from build123d import *

# Parameters (mm, degrees)
SKETCH_1_W          = 120
SKETCH_1_H          = 20
EXTRUDE_1_DEPTH     = 50
SKETCH_2_W          = 6
SKETCH_2_H          = 20
EXTRUDE_2_DEPTH     = 20
CUT_EXTRUDE_1_DEPTH = 114
SKETCH_4_R          = 2.6
SKETCH_4_W          = 20
SKETCH_4_H          = 20
CUT_EXTRUDE_2_DEPTH = 114
SKETCH_5_R          = 5
CUT_EXTRUDE_3_DEPTH = 3
CUT_EXTRUDE_4_DEPTH = 300
SKETCH_8_R          = 5
CUT_EXTRUDE_5_DEPTH = 300
SKETCH_9_R          = 5
SKETCH_9_R_2        = 2.6
EXTRUDE_3_DEPTH     = 3


with BuildPart() as part:
    # 草图1 → 凸台-拉伸1 (new body)
    with BuildSketch(Plane(origin=(0, 0, 0), x_dir=(1, 0, 0), z_dir=(0, 1, 0))):
        with Locations((60, 10)):
            Rectangle(SKETCH_1_W, SKETCH_1_H)
    extrude(amount=EXTRUDE_1_DEPTH)

    # 草图2 → 凸台-拉伸2 (add)
    with BuildSketch(Plane.XY):
        with Locations((3, -10)):
            Rectangle(SKETCH_2_W, SKETCH_2_H)
    extrude(amount=-EXTRUDE_2_DEPTH)

    # 草图3 → 切除-拉伸1 (cut)
    with BuildSketch(Plane(origin=(120, 0, 0), x_dir=(0, 0, -1), z_dir=(1, 0, 0))):
        Polygon((0, 50), (20, 0), (0, 0), align=None)
    extrude(amount=-CUT_EXTRUDE_1_DEPTH, mode=Mode.SUBTRACT)

    # 草图4 → 切除-拉伸2 (cut)
    with BuildSketch(Plane(origin=(6, 0, 0), x_dir=(0, 0, -1), z_dir=(1, 0, 0))):
        with Locations(Location((10, 10, 0), (0, 0, 90))):
            Circle(SKETCH_4_R)
        with Locations((10, -10)):
            Rectangle(SKETCH_4_W, SKETCH_4_H)
    extrude(amount=-CUT_EXTRUDE_2_DEPTH, mode=Mode.SUBTRACT)

    # 草图5 → 切除-拉伸3 (cut)
    with BuildSketch(Plane(origin=(6, 0, 0), x_dir=(0, 0, -1), z_dir=(1, 0, 0))):
        with Locations(Location((10, 10, 0), (0, 0, 90))):
            Circle(SKETCH_5_R)
    extrude(amount=-CUT_EXTRUDE_3_DEPTH, mode=Mode.SUBTRACT)

    # 草图6 → 切除-拉伸4 (cut)
    with BuildSketch(Plane(origin=(0, 50, 0), x_dir=(1, 0, 0), z_dir=(0, 1, 0))):
        with BuildLine():
            ThreePointArc((62.6, 10), (61.838477631, 11.838477631), (60, 12.6))
            Line((60, 12.6), (60, 7.4))
            ThreePointArc((60, 7.4), (61.838477631, 8.161522369), (62.6, 10))
        make_face()
        with BuildLine():
            Line((60, 7.4), (60, 12.6))
            ThreePointArc((60, 12.6), (57.4, 10), (60, 7.4))
        make_face()
    extrude(amount=-CUT_EXTRUDE_4_DEPTH, mode=Mode.SUBTRACT)

    # 草图8 → 切除-拉伸5 (cut)
    with BuildSketch(Plane(origin=(0, 50, 0), x_dir=(1, 0, 0), z_dir=(0, 1, 0))):
        with Locations(Location((60, 10, 0), (0, 0, 270))):
            Circle(SKETCH_8_R)
    extrude(amount=-CUT_EXTRUDE_5_DEPTH, mode=Mode.SUBTRACT)

    # 草图9 → 凸台-拉伸3 (add)
    with BuildSketch(Plane(origin=(0, 50, 0), x_dir=(1, 0, 0), z_dir=(0, 1, 0))):
        with Locations(Location((60, 10, 0), (0, 0, 270))):
            Circle(SKETCH_9_R)
        with Locations(Location((60, 10, 0), (0, 0, 270))):
            Circle(SKETCH_9_R_2, mode=Mode.SUBTRACT)
    extrude(amount=-EXTRUDE_3_DEPTH)


solid = part.part
Geometry: final body of the model. Coordinates: model frame, mm. A direction names the side the tool comes from. Round coordinates to 2 decimals unless told otherwise and drop trailing zeros. Loops run counter-clockwise (first coordinate to the right, second up) from the corner with the lowest first, then second, coordinate; pieces in that order, holes last.
Q1. Section B-B on x = 60. Return loops of the section in (y, z), plus the area to 3 significant figures.
Q2. Section A-A on z = -10. Return loops of the section in (x, y).
Q3. Pull-direction query (Z, two-part tool) for faces 1 (the flat face through (58, 47, -8)), 2 (the flat face through (59, 25, -20)), 3 (the cylindrical face through (60, 34, -15)), 4 (the flat face through (3, 0, -10)); classes: released by +Z, released by -Z, zero draft, split by the parting line, or undercut.
Q4. Pin query (flat end, axial travel): P1, Ø3, axis at x = 24.5, z = -8.5, coming from the -Y side; P2, Ø4, axis at x = 60, z = -10, coming from the -Y side; P3, Ø2, axis at x = 94, y = 30.5, coming from the +Z side; P4, Ø5, axis at x = 104.5, y = 37, coming from the +Z side. Return the tip coordinate at first contact, or that it passes through.
Q5. Material intervals for L1, parallel to X at y = 26, z = -10; L2, parallel to Z at x = 5, y = 10; L3, parallel to Z at x = 2.3, y = 10, sorted ascending.
Q6. Access query for faces 5 (the cylindrical face through (4.52, 14.77, -8.5)), 6 (the flat face through (6, 19, -5)), 7 (the flat face through (61, 50, -15)). Directions: +Z, -Z, +X, -X, +Y, -Y. A direction counts if a zero-diameter tool reaches every point of the face in a straight line with its end or side. Return the directions, or none.
Q7. Section C-C on y = 10. Return loops of the section in (x, z), plus the area to 3 significant figures.
Q8. Section D-D on z = -1.5. Return loops of the section in (x, y).
Evaluation:
1. outline: (0, -20) - (50, -20) - (50, -12.6) - (47, -12.6) - (47, -15) - (12.5, -15) - close; (37.5, -5) - (47, -5) - (47, -7.4) - (50, -7.4) - (50, 0) - close
1. area: 264 mm2
2. outline: (0, 0) - (6, 0) - (6, 5) - (3, 5) - (3, 7.4) - (0, 7.4) - close; (0, 12.6) - (3, 12.6) - (3, 15) - (6, 15) - (6, 25) - (55, 25) - (55, 47) - (57.4, 47) - (57.4, 50) - (0, 50) - close; (62.6, 47) - (65, 47) - (65, 25) - (120, 25) - (120, 50) - (62.6, 50) - close
3. face 1: undercut
3. face 2: released by -Z
3. face 3: undercut
3. face 4: zero draft
4. P1: stops at y = 25
4. P2: passes through
4. P3: stops at z = -7.4
4. P4: stops at z = -4.2
5. L1: x = 0 to 55, 65 to 120
5. L2: z = -20 to -15, -5 to 0
5. L3: z = -20 to -12.6, -7.4 to 0
6. face 5: +X
6. face 6: +Z, +X, -Y
6. face 7: +Z, -Z, +X, -X, +Y
7. outline: (0, -20) - (120, -20) - (120, -16) - (6, -16) - (6, -15) - (3, -15) - (3, -12.6) - (0, -12.6) - close; (0, -7.4) - (3, -7.4) - (3, -5) - (6, -5) - (6, 0) - (0, 0) - close
7. area: 530 mm2
8. outline: (0, 0) - (6, 0) - (6, 46.25) - (120, 46.25) - (120, 50) - (0, 50) - close
